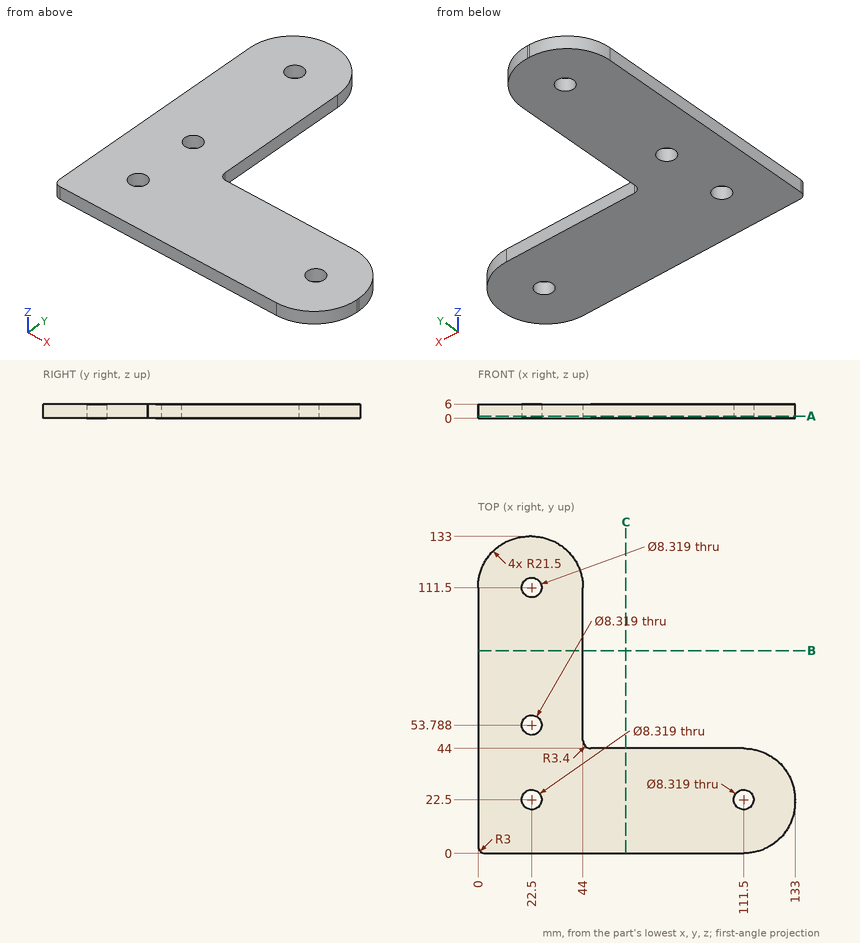
Check sheet for the drawn part. Datum: minimum x, y, z corner. Units: mm. Round coordinates to 2 decimals unless told otherwise and drop trailing zeros. Loops run counter-clockwise (first coordinate to the right, second up) from the corner with the lowest first, then second, coordinate; pieces in that order, holes last.
Item 1: Cross-section at A-A on z = 0.95. Record the boundary of the cut face in (x, y), then the cut area to 3 significant figures.
Item 2: Gauge pin test, flat ends, axial feed: pin 1 (3 mm diameter, centred on y = 77, z = 2, fed in from +X); pin 2 (1.5 mm diameter, centred on y = 115.5, z = 4, fed in from -X). Record the tip position at first contact, or that the pin passes through.
Item 3: Cross-section at B-B on y = 85. Record the boundary of the cut face in (x, z).
Item 4: Thickness scan on line 1 (Y direction, x = 107, z = 4); line 2 (Y direction, x = 111.5, z = 3.4); line 3 (Y direction, x = 24, z = 3.85). Record the ranges inside material, lowest first.
Answer sheet:
1. outline: (0, 3) arc R3 ccw to (3, 0) - (111.5, 0) arc R21.5 ccw to (133, 21.5) - (133, 22.5) arc R21.5 ccw to (111.5, 44) - (47.4, 44) arc R3.4 cw to (44, 47.4) - (44, 111.5) arc R21.5 ccw to (22.5, 133) - (21.5, 133) arc R21.5 ccw to (0, 111.5) - close; hole circle Ø8.32 at (22.5, 22.5); hole circle Ø8.32 at (22.5, 53.79); hole circle Ø8.32 at (22.5, 111.5); hole circle Ø8.32 at (111.5, 22.5)
1. area: 9,150 mm2
2. pin 1: stops at x = 44
2. pin 2: stops at x = 0.25
3. outline: (0, 0) - (44, 0) - (44, 6) - (0, 6) - close
4. line 1: y = 0 to 44
4. line 2: y = 0 to 18.34, 26.66 to 44
4. line 3: y = 0 to 18.62, 26.38 to 49.91, 57.67 to 107.62, 115.38 to 132.95
